Here's how the part is built. I have some questions about the finished solid (model axes, mm). Face numbers are marked on the shaded views. A direction names the side the tool comes from. Round coordinates to 2 decimals unless told otherwise and drop trailing zeros. Loops run counter-clockwise (first coordinate to the right, second up) from the corner with the lowest first, then second, coordinate; pieces in that order, holes last. Notation, with made-up numbers: M 12.25,32 L 39.25,32 A17 ccw 39.25,55 Z; hole C 26.5,14 d9. An arc over 180 degrees is marked long. Use a Markdown table: item, result.
Autodesk Inventor part; units mm, degrees
ref_plane "YZ Plane" through (0, 0, 0) normal (1, 0, 0) x (0, 1, 0)
ref_plane "XZ Plane" through (0, 0, 0) normal (0, 1, 0) x (-1, 0, 0)
ref_plane "XY Plane" through (0, 0, 0) normal (0, 0, 1) x (1, 0, 0)
sketch "Sketch2" plane through (0, 0, 0) normal (0, 1, 0) x (-1, 0, 0)
  line L0 (12.65, -2.45) -> (12.65, 2.45)
  line L1 (-12.65, 2.45) -> (-12.65, -2.45)
  line L2 (-12.65, -2.45) -> (12.65, 2.45) construction
  line L3 (12.65, -2.45) -> (-12.65, 2.45) construction
  line L4 (-2.45, -12.65) -> (2.45, -12.65)
  line L5 (2.45, 12.65) -> (-2.45, 12.65)
  line L6 (-2.45, -12.65) -> (2.45, 12.65) construction
  line L7 (2.45, -12.65) -> (-2.45, 12.65) construction
  line L8 (12.65, 2.45) -> (2.45, 2.45)
  line L9 (-2.45, 2.45) -> (-12.65, 2.45)
  line L10 (2.45, -12.65) -> (2.45, -2.45)
  line L11 (2.45, 2.45) -> (2.45, 12.65)
  line L12 (-12.65, -2.45) -> (-2.45, -2.45)
  line L13 (2.45, -2.45) -> (12.65, -2.45)
  line L14 (-2.45, 12.65) -> (-2.45, 2.45)
  line L15 (-2.45, -2.45) -> (-2.45, -12.65)
  circle A0 centre (0, 0) radius 1.5
  point P0 (0, 0)
  dimension "d7" = 4.9
  dimension "d8" = 4.9
  dimension "d9" = 10.2
  dimension "d10" = 3
extrude "Extrusion2" add sketch "Sketch2" along normal blind 1.9
fillet "Fillet1" radius 2.45 1 edges at (2.45, 0.95, 12.65)
fillet "Fillet2" radius 2.45 1 edges at (-2.45, 0.95, 12.65)
fillet "Fillet3" radius 2.45 1 edges at (12.65, 0.95, 2.45)
fillet "Fillet4" radius 2.45 1 edges at (12.65, 0.95, -2.45)
fillet "Fillet5" radius 2.45 1 edges at (2.45, 0.95, -12.65)
fillet "Fillet6" radius 2.45 1 edges at (-12.65, 0.95, 2.45)
fillet "Fillet7" radius 2.45 1 edges at (-12.65, 0.95, -2.45)
fillet "Fillet8" radius 2.45 1 edges at (-2.45, 0.95, -12.65)
chamfer "Chamfer1" distance 2 angle 45 1 edges at (-2.45, 0.95, -2.45)
chamfer "Chamfer2" distance 2 angle 45 1 edges at (2.45, 0.95, -2.45)
chamfer "Chamfer3" distance 2 angle 45 1 edges at (2.45, 0.95, 2.45)
chamfer "Chamfer4" distance 2 angle 45 1 edges at (-2.45, 0.95, 2.45)
equation "\"d7\" = ServoArmWidth"
equation "\"d8\" = ServoArmWidth"
equation "\"d9\" = ServoArmLength"
equation "\"d10\" = ServoArmHoleRequired"
equation "\"d11\" = ServoArmThickness"
equation "\"d13\" = ServoArmExternFillet"
equation "\"d14\" = ServoArmExternFillet"
equation "\"d15\" = ServoArmExternFillet"
equation "\"d16\" = ServoArmExternFillet"
equation "\"d17\" = ServoArmExternFillet"
equation "\"d18\" = ServoArmExternFillet"
equation "\"d19\" = ServoArmExternFillet"
equation "\"d20\" = ServoArmExternFillet"
equation "\"d21\" = ServoArmInternFillet"
equation "\"d24\" = ServoArmInternFillet"
equation "\"d27\" = ServoArmInternFillet"
equation "\"d30\" = ServoArmInternFillet"
equation "\"ServoArmWidth\" = 4.9"
equation "\"ServoArmSpacing\" = 0.2"
equation "\"ServoArmWidthRequired\" = ServoArmWidth + 2 * ServoArmSpacing"
equation "\"ServoArmLength\" = 10.2"
equation "\"ServoArmLengthRequired\" = ServoArmLength + 2 * ServoArmSpacing"
equation "\"ServoArmThickness\" = 1.9"
equation "\"ServoArmHoleRequired\" = 3"
equation "\"ServoArmInternFillet\" = 2"
equation "\"ServoArmExternFillet\" = 0.5 * ServoArmWidth"
equation "\"ServoArmHeadScrewTrace\" = 5.5"
equation "\"ServoArmHeadScrewThickness\" = 2.5"
properties part number "SimplifiedServoArm"
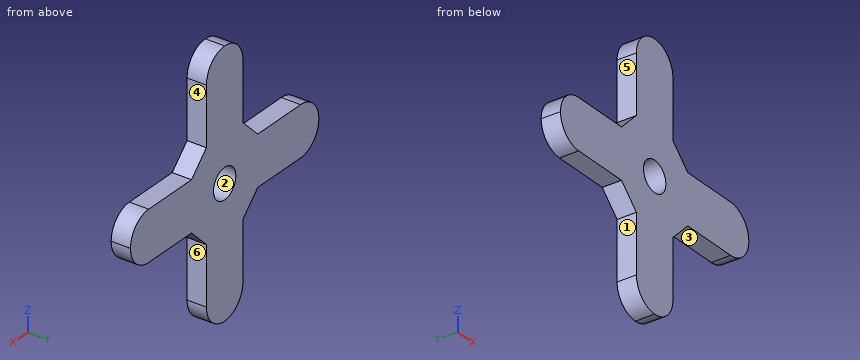
1. Imagine slicing it at B-B, the plane z = 1. Write out the boundary of the cut face in (x, y), then the cut area to 3 significant figures.
Answer sheet:
| item | result |
|---|---|
| outline | M -12.44,0 L -1.12,0 L -1.12,1.9 L -12.44,1.9 Z; M 1.12,0 L 12.44,0 L 12.44,1.9 L 1.12,1.9 Z |
| area | 43.0 mm2 |
2. Imagine slicing it at D-D, the plane x = -6.5. Write out the boundary of the cut face in (y, z), then the cut area to 3 significant figures.
Answer sheet:
| item | result |
|---|---|
| outline | M 0,-2.45 L 1.9,-2.45 L 1.9,2.45 L 0,2.45 Z |
| area | 9.31 mm2 |
3. We'd pull the mould along X, two halves only. Please class the marked faces 1, 2 and 3: +X half, -X half, draft (parallel to the pull), parting line (faces both ways), or undercut.
Answer sheet:
| item | result |
|---|---|
| face 1 | -X half |
| face 2 | undercut |
| face 3 | draft |
4. Imagine slicing it at C-C, the plane z = 4. Write out the boundary of the cut face in (x, y).
Answer sheet:
| item | result |
|---|---|
| outline | M -2.9,0 L 2.9,0 L 2.9,1.9 L -2.9,1.9 Z |
5. For pin 1 Ø0.6 at (y, z) = (0.5, -8) entering from +X; pin 2 Ø0.6 at (x, y) = (7.5, 1.5) entering from -Z; pin 3 Ø6 at (x, z) = (-5.5, -3.5) entering from -Y; pin 4 Ø1 at (y, z) = (1, 7.5) entering from -X, each with a flat end and sliding along its axis, tell me the tip position at first contact or that it passes through.
Answer sheet:
| item | result |
|---|---|
| pin 1 | x = 2.45 |
| pin 2 | z = -2.45 |
| pin 3 | y = 0 |
| pin 4 | x = -2.45 |
6. Which directions (+Z, -Z, +X, -X, +Y, -Y) give clear straight access to the entire face, cutting with the end or side of a thin tool? Please do the marked faces 4, 5 and 6.
Answer sheet:
| item | result |
|---|---|
| face 4 | +Z, +X, +Y, -Y |
| face 5 | +Z, -X, +Y, -Y |
| face 6 | -Z, +X, +Y, -Y |
7. I need wall thicknesses on probe 1 along Z at (x, y) = (0, 1.3); probe 2 along X at (y, z) = (0.85, 5.5); probe 3 along Z at (x, y) = (-1.25, 1.8). Which ranges of each line are inside material? Lowest first, please. Write a range as from..to.
Answer sheet:
| item | result |
|---|---|
| probe 1 | -12.65..-1.5, 1.5..12.65 |
| probe 2 | -2.45..2.45 |
| probe 3 | -12.31..-0.83, 0.83..12.31 |
